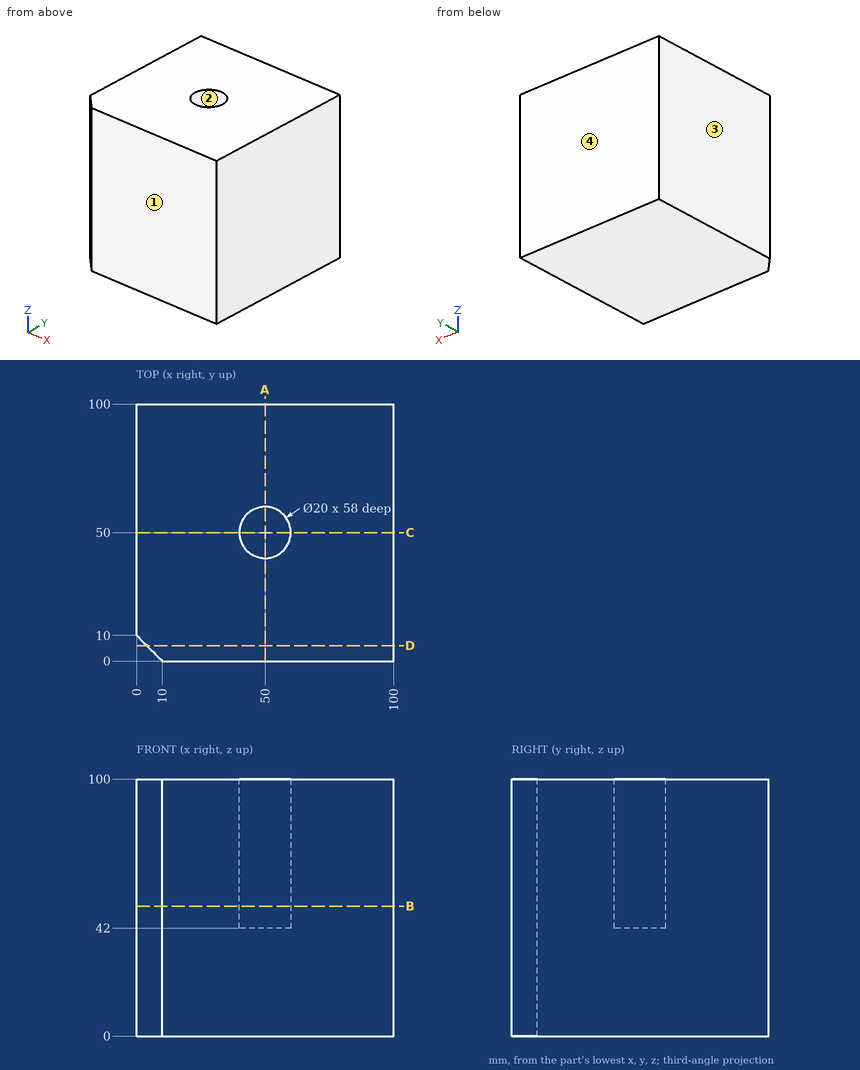
Could you check a few things on this drawing? It's one solid part, dimensions in mm from its lowest x, y, z. Round coordinates to 2 decimals unless told otherwise and drop trailing zeros. Order: outer loops, then holes, each group sorted by start corner. A loop starts at its lowest first (then second) coordinate and runs counter-clockwise, first axis right, second up. Notation, with made-up numbers: M 11.5,51.25 L 43.5,51.25 A24 ccw 43.5,64.25 Z; hole C 4,16.5 d3. An arc over 180 degrees is marked long. Use a Markdown table: item, result.
1) If we mould it in two halves opening along Y, with no side actions, what happens to the marked faces 1, 2, 3 and 4? For each: +Y half, -Y half, draft (parallel to the pull), parting line (faces both ways), or undercut.
Geometry says:
| item | result |
|---|---|
| face 1 | -Y half |
| face 2 | undercut |
| face 3 | draft |
| face 4 | +Y half |
2) Imagine slicing it at D-D (y = 6). List the corners of the cut face in (x, z) for me.
Geometry says:
| item | result |
|---|---|
| outline | M 4,0 L 100,0 L 100,100 L 4,100 Z |
3) If I drill on line 1 along Y through (x, z) = (50, 57); line 2 along X through (y, z) = (59, 50.5), over which ranges is the centre line in solid material (lowest first)?
Geometry says:
| item | result |
|---|---|
| line 1 | y = 0 to 40, 60 to 100 |
| line 2 | x = 0 to 45.64, 54.36 to 100 |
4) I'm going to push a flat-ended pin straight in: P1, Ø6, axis at y = 23.5, z = 18, coming from the -X side. Where does the tip first touch, or does it pass through?
Geometry says:
| item | result |
|---|---|
| P1 | stops at x = 0 |
5) Imagine slicing it at A-A (x = 50). List the corners of the cut face in (y, z) for me, then the cut area to 3 significant figures.
Geometry says:
| item | result |
|---|---|
| outline | M 0,0 L 100,0 L 100,100 L 60,100 L 60,42 L 40,42 L 40,100 L 0,100 Z |
| area | 8,840 mm² |
6) Imagine slicing it at B-B (z = 50.5). List the corners of the cut face in (x, y) for me, then the cut area to 3 significant figures.
Geometry says:
| item | result |
|---|---|
| outline | M 0,10 L 10,0 L 100,0 L 100,100 L 0,100 Z; hole C 50,50 d20 |
| area | 9,640 mm² |
